from build123d import *

# Parameters (mm, degrees)
TABAN_FLAN_1_DEPTH    = 25
IZIM9_W               = 9.15
IZIM9_H               = 35
KES_EKSTR_ZYON1_DEPTH = 32.162677998
IZIM11_R              = 2.6
KES_EKSTR_ZYON2_DEPTH = 10
RADYUS1_R             = 2.5


# Sheet-metal steps are written as plain solids
with BuildPart() as part:
    # Çizim1 → Taban-Flanş1 (new, symmetric)
    with BuildSketch(Plane.XY):
        with BuildLine():
            Line((-12.5, 0), (12.5, 0))
            ThreePointArc((12.5, 0), (14.537154879, -7.765591238), (8.95035213, -2))
            Line((8.95035213, -2), (10.233357384, -2.777108434))
            ThreePointArc((10.233357384, -2.777108434), (13.800833838, -6.458751031), (12.5, -1.5))
            Line((12.5, -1.5), (-12.5, -1.5))
            Line((-12.5, -1.5), (-12.5, 0))
        make_face()
    extrude(amount=TABAN_FLAN_1_DEPTH, both=True)

    # Çizim9 → Kes-Ekstrüzyon1 (cut, through all)
    with BuildSketch(Plane(origin=(0, 0, 0), x_dir=(1, 0, 0), z_dir=(0, 1, 0))):
        with Locations((12.075, 0)):
            Rectangle(IZIM9_W, IZIM9_H)
    extrude(amount=-KES_EKSTR_ZYON1_DEPTH, mode=Mode.SUBTRACT)

    # Çizim11 → Kes-Ekstrüzyon2 (cut)
    with BuildSketch(Plane(origin=(0, 0, 0), x_dir=(1, 0, 0), z_dir=(0, 1, 0))):
        with Locations(Location((-2.5, 15, 0), (0, 0, 180))):
            Circle(IZIM11_R)
        with Locations(Location((-2.5, -15, 0), (0, 0, 180))):
            Circle(IZIM11_R)
    extrude(amount=-KES_EKSTR_ZYON2_DEPTH, mode=Mode.SUBTRACT)

    # Radyus1
    radyus1_edges = [part.edges().sort_by_distance(p)[0] for p in [
        (-12.5, -0.75, 25),
        (-12.5, -0.75, -25),
    ]]
    fillet(radyus1_edges, radius=RADYUS1_R)


solid = part.part
Source: CAD feature listing. Evaluate the final solid. Frame: model axes, mm. A direction names the side the tool comes from. Round coordinates to 2 decimals unless told otherwise and drop trailing zeros. Loops run counter-clockwise (first coordinate to the right, second up) from the corner with the lowest first, then second, coordinate; pieces in that order, holes last.
Q1. Section C-C, the plane x = -2.5. Return loops of the section in (y, z).
Q2. Access query for faces 1 (the face through (9.58, -2.38, -21.2)), 2 (the face through (-12.5, -1, 0)), 3 (the face through (7.5, -1, 0)). Directions: +Z, -Z, +X, -X, +Y, -Y. A direction counts if a zero-diameter tool reaches every point of the face in a straight line with its end or side. Return the directions, or none.
Q3. Section B-B, the plane y = -4.15. Return loops of the section in (x, z), plus the area to 3 significant figures.
Q4. Mould query, pull axis Y, two halves, no side actions, for faces 4 (the face through (9.58, -2.38, 21.3)), 5 (the face through (-3, 0, 0)), 6 (the face through (6, -1, -25)). Classes: pulls with the +Y half, pulls with the -Y half, needs draft (parallel to the pull), parting line crosses it, or undercut.
Q5. Ray query, line 1 (Y direction, x = 12.5, z = -21.5); line 2 (Z direction, x = 14.25, y = -1); line 3 (X direction, y = -4.15, z = -19.75). Return the intervals inside material, ascending.
Q6. Section D-D, the plane x = 12. Return loops of the section in (y, z).
Q7. Section A-A, the plane z = -15. Return loops of the section in (x, y), plus the area to 3 significant figures.
Q8. First-contact query: P1, Ø7, axis at x = -2.5, z = 15, coming from the -Y side; P2, Ø0.8, axis at y = -1, z = -4.5, coming from the +X side; P3, Ø1.5, axis at x = 12.5, y = -2.5, coming from the +Z side. Flat tips, straight axial feed; report the tip coordinate or a pass-through.
Solutions:
1. outline: (-1.5, -25) - (0, -25) - (0, -17.6) - (-1.5, -17.6) - close; (-1.5, -12.4) - (0, -12.4) - (0, 12.4) - (-1.5, 12.4) - close; (-1.5, 17.6) - (0, 17.6) - (0, 25) - (-1.5, 25) - close
2. face 1: +Z, -Z
2. face 2: +Z, -Z, -X, +Y, -Y
2. face 3: +X, +Y, -Y
3. outline: (8.35, -25) - (9.85, -25) - (9.85, -17.5) - (8.35, -17.5) - close; (8.35, 17.5) - (9.85, 17.5) - (9.85, 25) - (8.35, 25) - close; (15.15, -25) - (16.65, -25) - (16.65, -17.5) - (15.15, -17.5) - close; (15.15, 17.5) - (16.65, 17.5) - (16.65, 25) - (15.15, 25) - close
3. area: 45.0 mm2
4. face 4: undercut
4. face 5: pulls with the +Y half
4. face 6: needs draft
5. line 1: y = -8.3 to -6.8, -1.5 to 0
5. line 2: z = -25 to -17.5, 17.5 to 25
5. line 3: x = 8.35 to 9.85, 15.15 to 16.65
6. outline: (-8.27, -25) - (-6.75, -25) - (-6.75, -17.5) - (-8.27, -17.5) - close; (-8.27, 17.5) - (-6.75, 17.5) - (-6.75, 25) - (-8.27, 25) - close; (-1.5, -25) - (0, -25) - (0, -17.5) - (-1.5, -17.5) - close; (-1.5, 17.5) - (0, 17.5) - (0, 25) - (-1.5, 25) - close
7. outline: (-12.5, -1.5) - (-5.1, -1.5) - (-5.1, 0) - (-12.5, 0) - close; (0.1, -1.5) - (7.5, -1.5) - (7.5, 0) - (0.1, 0) - close
7. area: 22.2 mm2
8. P1: stops at y = -1.5
8. P2: stops at x = 7.5
8. P3: passes through
